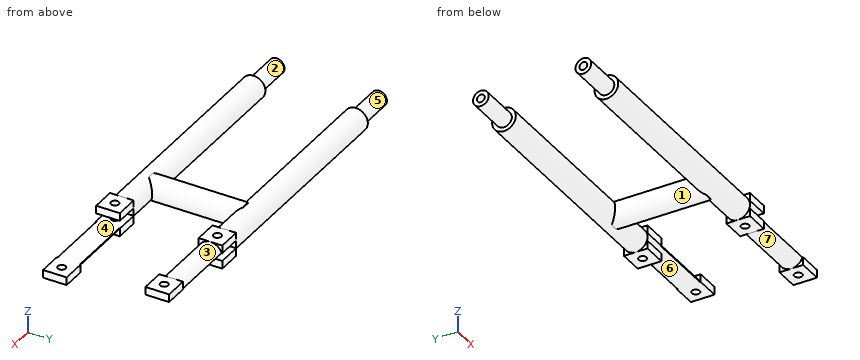
from build123d import *

# Parameters (mm, degrees)
F1_DEPTH      = 15
F2_R          = 7.5
F3_DEPTH      = 240
F4_R          = 7.5
F5_DEPTH      = 30
F5_DEPTH_BACK = 30
F6_W          = 15
F6_H          = 15
F7_DEPTH      = 15
F9_DEPTH      = 40.1
F11_DEPTH     = 54.1
F12_R         = 2.5
F13_DEPTH     = 25
F15_R         = 2.5
F16_DEPTH     = 25
F18_DEPTH     = 25
F17_R         = 7.5
F17_R_2       = 5
F19_DEPTH     = 25


# Not quite as in the source:
# - a feature names something its author has since deleted; it is built from what else it names


with BuildPart() as f1:
    # F0 (on Top) → F1 (new body)
    with BuildSketch(Plane.XY):
        Polygon((-240, -25), (-240, -40), (0, -40), (0, -25), (-100, -25), (-100, 25), (0, 25), (0, 40), (-240, 40), (-240, 25), (-115, 25), (-115, -25), align=None)
    extrude(amount=F1_DEPTH)

    # F2 (on Right) → F3 (intersect)
    with BuildSketch(Plane.YZ):
        with Locations((-32.5, 7.5)):
            Circle(F2_R)
        with Locations((32.5, 7.5)):
            Circle(F2_R)
    extrude(amount=-F3_DEPTH, mode=Mode.INTERSECT)

    # F4 (on Front) → F5 (join, two sides)
    with BuildSketch(Plane.XZ) as f5_sk:
        with Locations((-100, 7.5)):
            Circle(F4_R)
    extrude(amount=F5_DEPTH)
    extrude(f5_sk.sketch, amount=-F5_DEPTH_BACK)

    # F6 (on Top) → F7 (join)
    with BuildSketch(Plane.XY):
        with Locations((-65, 32.5)):
            Rectangle(F6_W, F6_H)
        with Locations((-65, -32.5)):
            Rectangle(F6_W, F6_H)
        with Locations((-7.5, 32.5)):
            Rectangle(F6_W, F6_H)
        with Locations((-7.5, -32.5)):
            Rectangle(F6_W, F6_H)
    extrude(amount=F7_DEPTH)

    # F8 (on Front) → F9 (cut)
    with BuildSketch(Plane.XZ):
        Polygon((0, 0), (0, 10), (-72.5, 10), (-72.5, 5), (-57.5, 5), (-57.5, 0), align=None)
    extrude(amount=-F9_DEPTH, mode=Mode.SUBTRACT)

    # F10 (on Front) → F11 (cut)
    with BuildSketch(Plane.XZ):
        Polygon((0, 5), (0, 15), (-57.5, 15), (-57.5, 10), (-72.5, 10), (-72.5, 5), (-57.5, 5), align=None)
    extrude(amount=F11_DEPTH, mode=Mode.SUBTRACT)

    # F12 (on Top) → F13 (cut)
    with BuildSketch(Plane.XY):
        with Locations((-65, 32.5)):
            Circle(F12_R)
        with Locations((-65, -32.5)):
            Circle(F12_R)
        with Locations((-7.5, -32.5)):
            Circle(F12_R)
        with Locations((-7.5, 32.5)):
            Circle(F12_R)
    extrude(amount=F13_DEPTH, mode=Mode.SUBTRACT)

    # F15 (on offset) → F16 (cut)
    with BuildSketch(Plane(origin=(-240, 0, 0), x_dir=(0, -1, 0), z_dir=(-1, 0, 0))):
        with Locations((-32.5, 7.5)):
            Circle(F15_R)
        with Locations((32.5, 7.5)):
            Circle(F15_R)
    extrude(amount=-F16_DEPTH, mode=Mode.SUBTRACT)

    # F0 (on Top) → F18 (cut)
    with BuildSketch(Plane.XY):
        Polygon((-240, -25), (-240, -40), (0, -40), (0, -25), (-100, -25), (-100, 25), (0, 25), (0, 40), (-240, 40), (-240, 25), (-115, 25), (-115, -25), align=None)
    extrude(amount=-F18_DEPTH, mode=Mode.SUBTRACT)

    # F17 (on offset) → F19 (cut)
    with BuildSketch(Plane(origin=(-240, 0, 0), x_dir=(0, -1, 0), z_dir=(-1, 0, 0))):
        with Locations((-32.5, 7.5)):
            Circle(F17_R)
        with Locations((-32.5, 7.5)):
            Circle(F17_R_2, mode=Mode.SUBTRACT)
        with Locations((32.5, 7.5)):
            Circle(F17_R)
        with Locations((32.5, 7.5)):
            Circle(F17_R_2, mode=Mode.SUBTRACT)
    extrude(amount=-F19_DEPTH, mode=Mode.SUBTRACT)


solid = f1.part
Verification items for the finished model (mm, model axes). Face numbers are marked on the shaded views. A direction names the side the tool comes from. Give positions to 0.01 mm unless a question says otherwise; leave off trailing zeros. Loops run counter-clockwise (first coordinate to the right, second up) from the corner with the lowest first, then second, coordinate; pieces in that order, holes last. Notation, with made-up numbers: (56.25, 72) - (108.25, 72) arc R27 ccw to (108.25, 100) - close; hole circle Ø5 at (33, -35.75). An arc over 180 degrees is marked (long way). Write item = value, one per line. Start each with the question number.
Q1. Cross-section at B-B, the plane z = 7.5. Enter the section's corners in (x, y), and give its area (4 significant figures).
Q2. Cross-section at C-C, the plane x = -100. Enter the section's corners in (y, z).
Q3. Thickness scan on line 1 (X direction, y = 32, z = 11.5); line 2 (Y direction, x = -65, z = 3.3); line 3 (Z direction, x = -231.5, y = -32.5). Record the ranges inside material, lowest first.
Q4. Depth check by flat-ended pin: P1, Ø4, axis at y = 32.5, z = 7.5, coming from the +X side; P2, Ø3, axis at x = -137, z = 4, coming from the -Y side; P3, Ø5, axis at x = -182, z = 13, coming from the -Y side. Enter the tip coordinate at first touch or a pass-through.
Q5. Tool access check on the marked faces 1, 2, 3 and 4. Record the directions out of +Z, -Z, +X, -X, +Y, -Y that give a thin tool (end or side, any length) a straight path to the whole face; none if there is none.
Q6. Cross-section at D-D, the plane x = -177.5. Enter the section's corners in (y, z), and give its area (3 significant figures).
Q7. Mould release check, pull along Y, two halves, no side actions. Record for the marked faces 5, 6 and 7: released by +Y, released by -Y, zero draft, split by the parting line, or undercut.
Q8. Cross-section at A-A, the plane x = -7.5. Enter the section's corners in (y, z).
Answer key:
q1.outline = (-240, -37.5) - (-215, -37.5) - (-215, -40) - (-72.5, -40) - (-72.5, -25) - (-92.5, -25) - (-92.5, 25) - (-72.5, 25) - (-72.5, 40) - (-215, 40) - (-215, 37.5) - (-240, 37.5) - (-240, 35) - (-215, 35) - (-215, 30) - (-240, 30) - (-240, 27.5) - (-215, 27.5) - (-215, 25) - (-107.5, 25) - (-107.5, -25) - (-215, -25) - (-215, -27.5) - (-240, -27.5) - (-240, -30) - (-215, -30) - (-215, -35) - (-240, -35) - close
q1.area = 5,275 mm^2
q2.outline = (-30, 0) - (30, 0) - (30, 0.43) arc R7.5 ccw (long way) to (30, 14.57) - (30, 15) - (-30, 15) - (-30, 14.57) arc R7.5 ccw (long way) to (-30, 0.43) - close
q3.line_1 = -240 to -67.45, -62.55 to -9.95, -5.05 to 0
q3.line_2 = -40 to -35, -30 to -25, 25 to 30, 35 to 40
q3.line_3 = 2.5 to 5, 10 to 12.5
q4.P1 = -72.5
q4.P2 = -39.73
q4.P3 = -39.37
q5.face_1 = none
q5.face_2 = -X
q5.face_3 = +Z
q5.face_4 = +X, +Y, -Y
q6.outline = circle Ø15 at (-32.5, 7.5); circle Ø15 at (32.5, 7.5)
q6.area = 353 mm^2
q7.face_5 = undercut
q7.face_6 = zero draft
q7.face_7 = split by the parting line
q8.outline = (-40, 0) - (-35, 0) - (-35, 5) - (-40, 5) - close; (-30, 0) - (-25, 0) - (-25, 5) - (-30, 5) - close; (25, 10) - (30, 10) - (30, 15) - (25, 15) - close; (35, 10) - (40, 10) - (40, 15) - (35, 15) - close
